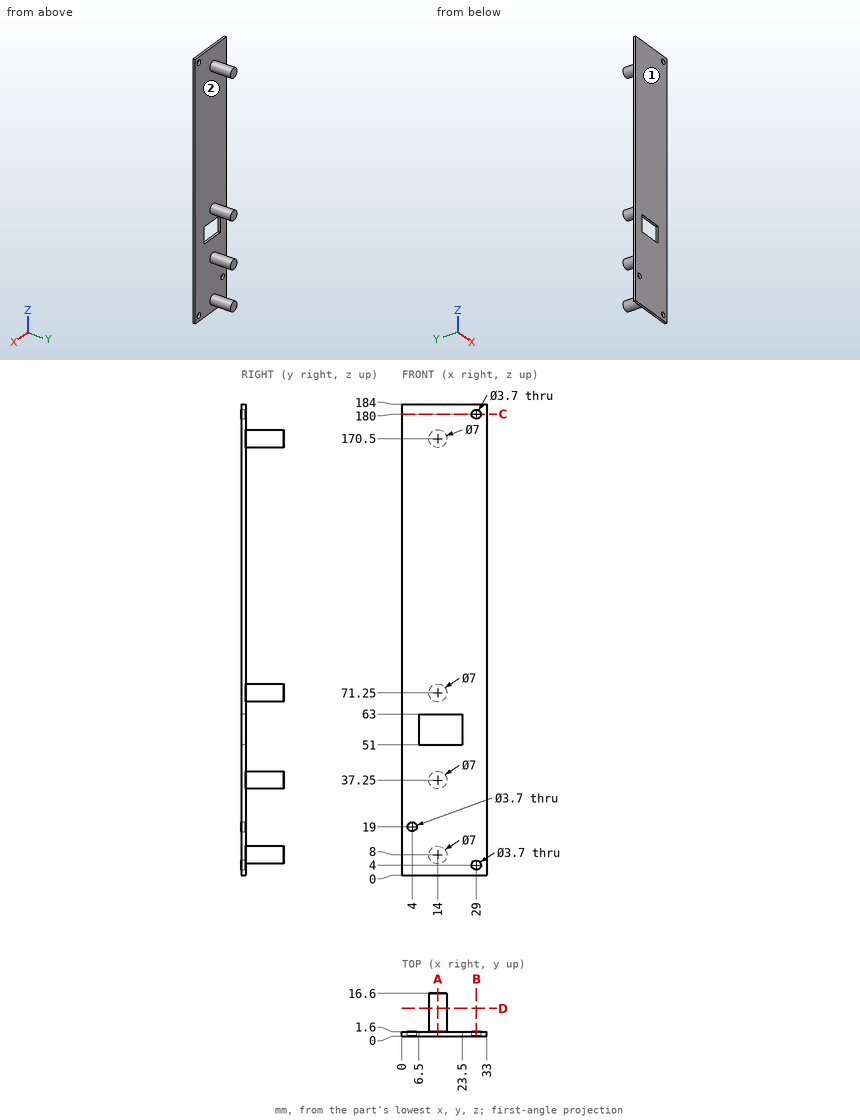
Could you check a few things on this drawing? It's one solid part, dimensions in mm from its lowest x, y, z. A direction names the side the tool comes from. Round coordinates to 2 decimals unless told otherwise and drop trailing zeros. Loops run counter-clockwise (first coordinate to the right, second up) from the corner with the lowest first, then second, coordinate; pieces in that order, holes last.
Q1. I want a section at A-A (x = 14). Write out the boundary of the cut face in (y, z).
Q2. Please list where these lines run through material, in increasing order: L1, parallel to X at y = 1.25, z = 19; L2, parallel to X at y = 0.5, z = 180; L3, parallel to Z at x = 15, y = 4.5.
Q3. For P1, Ø10, axis at x = 11.5, z = 104.5, coming from the +Y side; P2, Ø5, axis at x = 15, y = 8, coming from the -Z side, each with a flat end and sliding along its axis, tell me the tip position at first contact or that it passes through.
Q4. On a 3-axis mill with a long thin cutter (end or side, diameter ignored), from which of +Z, -Z, +X, -X, +Y, -Y can I reach the whole of each face in a straight line? I mean the marked faces 1 and 2. Say none if no direction works.
Q5. I want a section at C-C (z = 180). Write out the boundary of the cut face in (x, y).
Q6. I want a section at D-D (y = 10.75). Write out the boundary of the cut face in (x, z), and give its area (3 significant figures).
Q7. I want a section at B-B (x = 29). Write out the boundary of the cut face in (y, z).
Answer below:
1. outline: (0, 0) - (1.6, 0) - (1.6, 4.5) - (16.6, 4.5) - (16.6, 11.5) - (1.6, 11.5) - (1.6, 33.75) - (16.6, 33.75) - (16.6, 40.75) - (1.6, 40.75) - (1.6, 51) - (0, 51) - close; (0, 63) - (1.6, 63) - (1.6, 67.75) - (16.6, 67.75) - (16.6, 74.75) - (1.6, 74.75) - (1.6, 167) - (16.6, 167) - (16.6, 174) - (1.6, 174) - (1.6, 184) - (0, 184) - close
2. L1: x = 0 to 2.15, 5.85 to 33
2. L2: x = 0 to 27.15, 30.85 to 33
2. L3: z = 4.65 to 11.35, 33.9 to 40.6, 67.9 to 74.6, 167.15 to 173.85
3. P1: stops at y = 1.6
3. P2: stops at z = 4.5
4. face 1: +Z, -Z, +X, -X, -Y
4. face 2: +Y
5. outline: (0, 0) - (27.15, 0) - (27.15, 1.6) - (0, 1.6) - close; (30.85, 0) - (33, 0) - (33, 1.6) - (30.85, 1.6) - close
6. outline: circle Ø7 at (14, 8); circle Ø7 at (14, 37.25); circle Ø7 at (14, 71.25); circle Ø7 at (14, 170.5)
6. area: 154 mm2
7. outline: (0, 0) - (1.6, 0) - (1.6, 2.15) - (0, 2.15) - close; (0, 5.85) - (1.6, 5.85) - (1.6, 178.15) - (0, 178.15) - close; (0, 181.85) - (1.6, 181.85) - (1.6, 184) - (0, 184) - close
